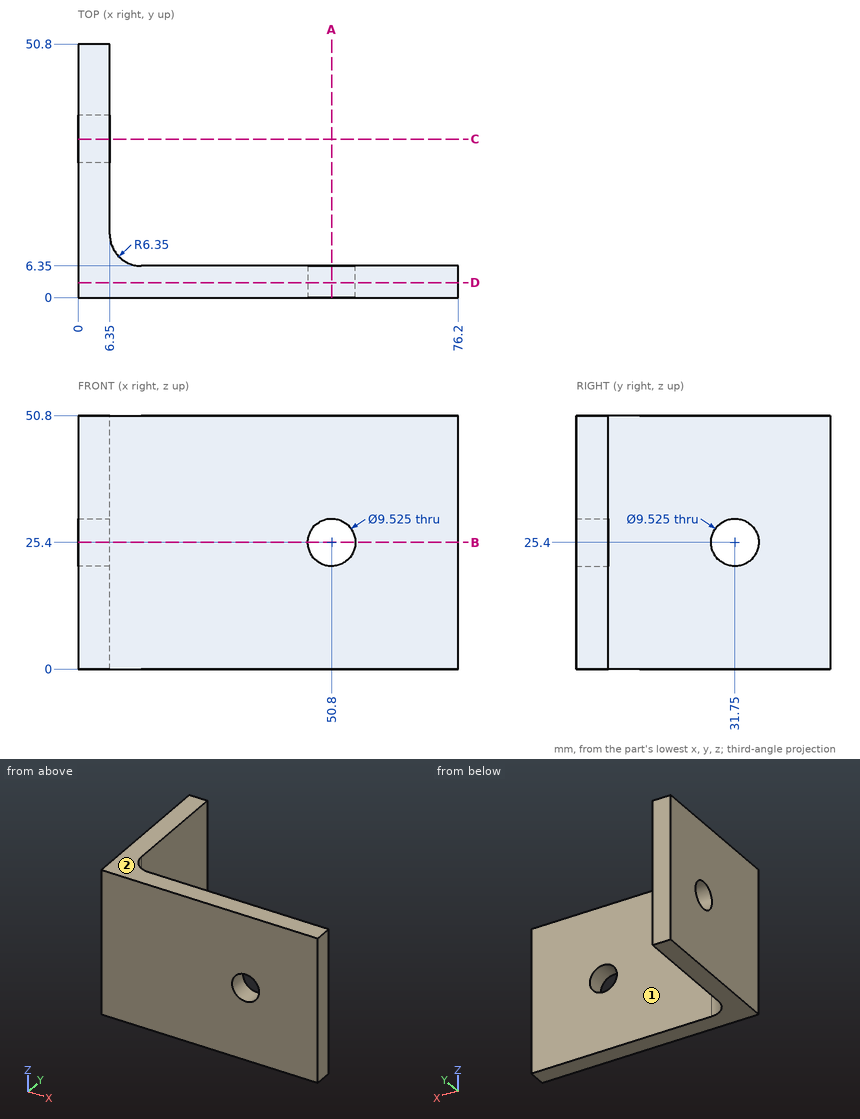
Job drawing, mm, ordinate dimensions from the low corner. One solid piece. A direction names the side the tool comes from. Coordinates: 2 decimals unless noted, no trailing zeros. Write each loop counter-clockwise with the first axis right and the second up, starting at its lowest first coordinate (ties: lowest second). Pieces come first, ordered by that corner, then holes.
Item 1: Slice it at D-D (y = 3). Write the cut outline in (x, z) (1 decimal).
Item 2: Which spindle directions (+Z, -Z, +X, -X, +Y, -Y) get a long thin tool onto all of the face, cutting with end or side? Do the marked faces 1 and 2. Say none if no direction does.
Item 3: Slice it at B-B (z = 25.4). Write the cut outline in (x, y), and give its area (3 significant figures).
Item 4: Pin check, flat tips, straight feed: pin 1 (1 mm diameter, centred on x = 40, z = 10.5, fed in from +Y); pin 2 (6 mm diameter, centred on y = 18, z = 17.5, fed in from +X); pin 3 (1 mm diameter, centred on x = 7.5, z = 12.5, fed in from +Y). Stop position of each tip, or through.
Item 5: Slice it at A-A (x = 50.8). Write the cut outline in (y, z), and give its area (3 significant figures).
Item 6: Probe line 1 (Y direction, x = 1.5, z = 25.4); line 2 (Z direction, x = 50.8, y = 4.25); line 3 (Y direction, x = 38, z = 45). List the from-to ranges inside material, lowest first.
Results found:
1. outline: (0, 0) - (76.2, 0) - (76.2, 50.8) - (0, 50.8) - close; hole circle Ø9.5 at (50.8, 25.4)
2. face 1: +Z, -Z, +X, +Y
2. face 2: +Z, +X, -X, +Y, -Y
3. outline: (0, 0) - (46.04, 0) - (46.04, 6.35) - (12.7, 6.35) arc R6.35 cw to (6.35, 12.7) - (6.35, 26.99) - (0, 26.99) - close; (0, 36.51) - (6.35, 36.51) - (6.35, 50.8) - (0, 50.8) - close; (55.56, 0) - (76.2, 0) - (76.2, 6.35) - (55.56, 6.35) - close
3. area: 654 mm2
4. pin 1: stops at y = 6.35
4. pin 2: stops at x = 6.35
4. pin 3: stops at y = 9.9
5. outline: (0, 0) - (6.35, 0) - (6.35, 20.64) - (0, 20.64) - close; (0, 30.16) - (6.35, 30.16) - (6.35, 50.8) - (0, 50.8) - close
5. area: 262 mm2
6. line 1: y = 0 to 26.99, 36.51 to 50.8
6. line 2: z = 0 to 20.64, 30.16 to 50.8
6. line 3: y = 0 to 6.35
